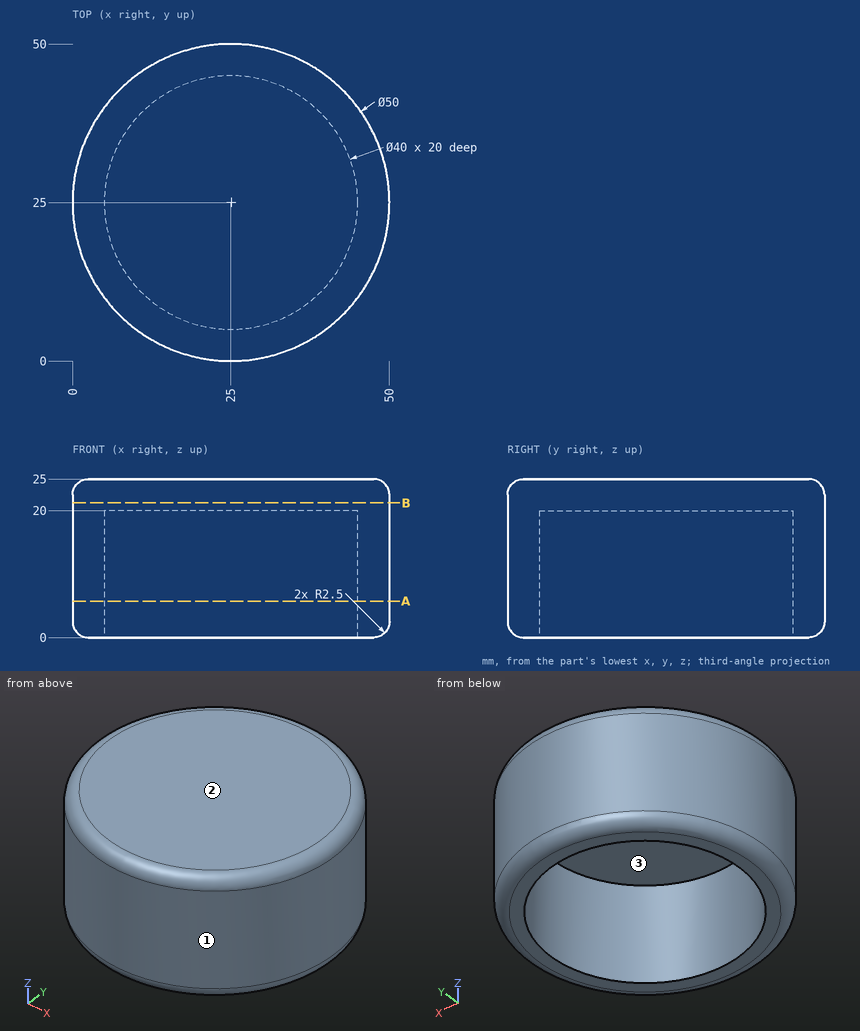
Study the drawing (mm; zero at the part's minimum x, y, z) and answer. Coordinates: 2 decimals unless noted, no trailing zeros. Write each loop counter-clockwise with the first axis right and the second up, starting at its lowest first coordinate (ties: lowest second). Pieces come first, ordered by that corner, then holes. Notation, with made-up numbers: (-40, 33) -> (-18, 33) arc R10 cw to (-18, 37) -> close; hole circle Ø11 at (-11.5, 21). An arc over 180 degrees is marked (long way). Write item = value, one per line.
(1) Section A-A on z = 5.75 is taken. Write down the section's boundary in (x, y), plus the area to 3 significant figures.
From the geometry:
outline = circle Ø50 at (25, 25); hole circle Ø40 at (25, 25)
area = 707 mm2
(2) Given pin 1 Ø12 at (y, z) = (39.5, 3.5) entering from -X; pin 2 Ø10 at (x, z) = (10.5, 13.5) entering from +Y; pin 3 Ø24 at (x, y) = (25, 25) entering from -Z, each flat-ended and moving along its own axis, determine where each tip first touches the part or whether it passes through.
From the geometry:
pin_1 = 1.49
pin_2 = 48.12
pin_3 = 20
(3) Straight lines are drawn through the part: L1, parallel to Z at x = 10.5, y = 24; L2, parallel to X at y = 10.5, z = 11.75; L3, parallel to X at y = 34.5, z = 3. For each, find the intervals that lie inside material, in ascending order. Write a range as from..to.
From the geometry:
L1 = 20..25
L2 = 4.63..11.23, 38.77..45.37
L3 = 1.88..7.4, 42.6..48.12
(4) Section B-B on z = 21.25 is taken. Write down the section's boundary in (x, y).
From the geometry:
outline = circle Ø50 at (25, 25)
(5) For a pull along X with two mould halves and no side action, classify the marked faces 1, 2 and 3 as +X half, -X half, draft (parallel to the pull), parting line (faces both ways), or undercut.
From the geometry:
face_1 = parting line
face_2 = draft
face_3 = undercut
